```python
from build123d import *

# Parameters (mm, degrees)
SKETCH1_R               = 25
BOSS_EXTRUDE1_DEPTH     = 900
SKETCH2_W               = 3
SKETCH2_H               = 10
CUT_EXTRUDE1_DEPTH      = 1
CUT_EXTRUDE1_DEPTH_BACK = 901
FILLET1_R               = 1


with BuildPart() as part:
    # Sketch1 → Boss-Extrude1 (new body)
    with BuildSketch(Plane.XY):
        Circle(SKETCH1_R)
    extrude(amount=BOSS_EXTRUDE1_DEPTH)

    # Sketch2 → Cut-Extrude1 (cut, two sides)
    with BuildSketch(Plane.XY.offset(900)) as cut_extrude1_sk:
        with Locations((0, 25)):
            Rectangle(SKETCH2_W, SKETCH2_H)
    extrude(amount=CUT_EXTRUDE1_DEPTH, mode=Mode.SUBTRACT)
    extrude(cut_extrude1_sk.sketch, amount=-CUT_EXTRUDE1_DEPTH_BACK, mode=Mode.SUBTRACT)

    # Fillet1
    fillet1_edges = [part.edges().sort_by_distance(p)[0] for p in [
        (1.5, 22.477479713, 900),
        (0, 20, 0),
        (-1.5, 22.477479713, 900),
        (-17.139136501, -18.200274723, 0),
        (-1.5, 22.477479713, 0),
        (-17.139136501, -18.200274723, 900),
        (1.5, 22.477479713, 0),
        (1.5, 24.954959427, 450),
        (0, 20, 900),
        (-1.5, 24.954959427, 450),
    ]]
    fillet(fillet1_edges, radius=FILLET1_R)


solid = part.part
```
Input: part model. Units: mm. Frame: model coordinates. Give positions to 0.01 mm unless a question says otherwise; leave off trailing zeros. Order: outer loops, then holes, each group sorted by start corner. A loop starts at its lowest first (then second) coordinate and runs counter-clockwise, first axis right, second up. Notation, with made-up numbers: M 44.5,-24.75 L 53.5,-24.75 A13 cw 53.5,-9.75 Z; hole C 77.25,-1.5 d6. An arc over 180 degrees is marked long. One line per question, with ' | ' between items.
1) Ray query, L1, parallel to X at y = 21, z = 190; L2, parallel to X at y = 2, z = 617; L3, parallel to Z at x = -2, y = 21.5. Return the intervals inside material, ascending.
Filled in:
L1: x = -13.56 to -1.5, 1.5 to 13.56 | L2: x = -24.92 to 24.92 | L3: z = 0.13 to 899.87
2) Section A-A on z = 770. Output: boundary loops of the cut face in (x, y), and give its area (3 significant figures).
Filled in:
outline: M -2.6,24.86 A25 ccw long 2.6,24.86 A1 ccw 1.5,23.87 L 1.5,20 L -1.5,20 L -1.5,23.87 A1 ccw Z | area: 1,950 mm2
3) Contact query for flat-ended pins moving along their axis: P1, Ø3, axis at y = 22.5, z = 564, coming from the -X side; P2, Ø12, axis at y = -14.5, z = 672.5, coming from the +X side; P3, Ø2, axis at y = 14, z = 374.5, coming from the +X side. Output: stop coordinate, or through.
Filled in:
P1: stops at x = -13.56 | P2: stops at x = 23.51 | P3: stops at x = 21.35
